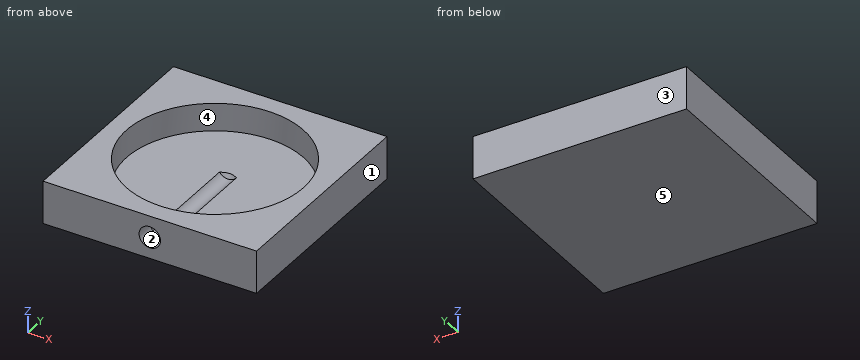
from build123d import *

# Parameters (mm, degrees)
F0_W     = 63.5
F0_H     = 12.7
F1_DEPTH = 63.5
F2_R     = 26.289
F3_DEPTH = 8.255
F5_D     = 6.35
F5_DEPTH = 38.1
F5_TIP   = 1.9077324654


with BuildPart() as f1:
    # F0 (on Front) → F1 (new body)
    with BuildSketch(Plane.XZ):
        with Locations((-24.3473223271, 6.35)):
            Rectangle(F0_W, F0_H)
    extrude(amount=F1_DEPTH)

    # F2 (on face) → F3 (cut)
    with BuildSketch(Plane.XY.offset(12.7)):
        with Locations((-24.3473223271, -31.75)):
            Circle(F2_R)
    extrude(amount=-F3_DEPTH, mode=Mode.SUBTRACT)

    # F5
    with Locations(Plane.XZ.offset(63.5)):
        with Locations((-24.3473223271, 6.35)):
            Hole(F5_D / 2, depth=F5_DEPTH)
            with Locations((0, 0, -(F5_DEPTH + F5_TIP / 2))):  # 118° drill point
                Cone(0, F5_D / 2, F5_TIP, mode=Mode.SUBTRACT)


solid = f1.part
The listing builds one solid part. Answer for the finished solid, in the listing's coordinates (mm). Face numbers are marked on the shaded views. A direction names the side the tool comes from. Give positions to 0.01 mm unless a question says otherwise; leave off trailing zeros. Loops run counter-clockwise (first coordinate to the right, second up) from the corner with the lowest first, then second, coordinate; pieces in that order, holes last.
Item 1: A cutting plane is placed at A-A (y = -31.75). Give the vertices of the cut face in (x, z) (3 decimals), then the cut area to 3 significant figures.
Derived:
outline: (-56.097, 0) - (7.403, 0) - (7.403, 12.7) - (1.942, 12.7) - (1.942, 4.445) - (-21.807, 4.445) arc R3.175 cw to (-26.887, 4.445) - (-50.636, 4.445) - (-50.636, 12.7) - (-56.097, 12.7) - close
area: 368 mm2
Item 2: A cutting plane is placed at D-D (y = -51). Give the vertices of the cut face in (x, z) (3 decimals), then the cut area to 3 significant figures.
Derived:
outline: (-56.097, 0) - (7.403, 0) - (7.403, 12.7) - (-6.443, 12.7) - (-6.443, 4.445) - (-21.807, 4.445) arc R3.175 cw to (-26.887, 4.445) - (-42.251, 4.445) - (-42.251, 12.7) - (-56.097, 12.7) - close
area: 506 mm2
Item 3: A cutting plane is placed at C-C (z = 6.35). Give the vertices of the cut face in (x, y), then the cut area to 3 significant figures.
Derived:
outline: (-56.1, -63.5) - (-27.52, -63.5) - (-27.52, -57.85) arc R26.29 cw (long way) to (-21.17, -57.85) - (-21.17, -63.5) - (7.4, -63.5) - (7.4, 0) - (-56.1, 0) - close
area: 1,830 mm2
Item 4: Determine the mould class of the marked faces 1, 2 and 3 for opening direction X: +X half, -X half, draft (parallel to the pull), parting line (faces both ways), or undercut.
Derived:
face 1: +X half
face 2: undercut
face 3: draft
Item 5: A cutting plane is placed at B-B (x = -39). Give the vertices of the cut face in (y, z) (3 decimals).
Derived:
outline: (-63.5, 0) - (0, 0) - (0, 12.7) - (-9.923, 12.7) - (-9.923, 4.445) - (-53.577, 4.445) - (-53.577, 12.7) - (-63.5, 12.7) - close
Item 6: Find the intervals of material crossed by line 1 along Y through (x, z) = (-25, 11); line 2 along X through (y, z) = (-31.75, 6.75); line 3 along Z through (x, y) = (-15.5, -46) (3 decimals), in increasing order.
Derived:
line 1: y = -63.5 to -58.03, -5.47 to 0
line 2: x = -56.1 to -50.64, 1.94 to 7.4
line 3: z = 0 to 4.445
Item 7: A tool of negligible diameter and unlimited length cuts with its end or side. For the marked faces 4 and 5, from which of +Z, -Z, +X, -X, +Y, -Y can it reach the whole face along a straight path? Write none if from no direction.
Derived:
face 4: +Z
face 5: -Z, +X, -X, +Y, -Y
